Check sheet for the modelled part. Datum: model origin and axes. Units: mm. A direction names the side the tool comes from. Give positions to 0.01 mm unless a question says otherwise; leave off trailing zeros. Loops run counter-clockwise (first coordinate to the right, second up) from the corner with the lowest first, then second, coordinate; pieces in that order, holes last. Notation, with made-up numbers: (-6.75, -12) - (29.25, -12) arc R7 cw to (29.25, -1) - close; hole circle Ø2 at (47.25, 38.5). An arc over 180 degrees is marked (long way). Answer in a Markdown table with one row per item. Add a question column.
(1) Go/stop test with flat-tipped pins: P1, Ø1.9, axis at y = 24.5, z = 3, coming from the -X side; P2, Ø1.9, axis at y = 22, z = 4.5, coming from the +X side; P3, Ø1.9, axis at x = -79, z = 2, coming from the +Y side. Record where each tip stops, or that it passes through.
(2) Sectioned sample at B-B on y = 18.5. Enter the section's corners in (x, z) (3 decimals).
(3) Draft check along X on faces 5 (the face through (-76.325, 15, 3)), 6 (the face through (40, -26.35, 3)), 7 (the face through (10, -23, 3)), 8 (the face through (-30, 23, 3)). Enter one of: released by +X, released by -X, zero draft, split by the parting line, or undercut.
(4) Sectioned sample at A-A on x = 67. Enter the section's corners in (y, z).
(5) Thickness scan on L1, parallel to X at y = 20.5, z = 4.5; L2, parallel to X at y = 19, z = 3.5 (3 decimals); L3, parallel to Y at x = -60, z = 2. Record the ranges inside material, lowest first.
(6) Set-up check for faces 1 (the face through (-80, 10, 3)), 2 (the face through (63, 20, 3)), 3 (the face through (76.325, -15, 3)), 4 (the face through (30, 23, 3)): record each of +Z, -Z, +X, -X, +Y, -Y from which the full face is reachable in a straight line by a thin tool's end or side.
from build123d import *

# Parameters (mm, degrees)
ESQUISSE1_W             = 165.35
ESQUISSE1_H             = 52.7
BOSS_EXTRU_1_DEPTH      = 6.35
ESQUISSE3_W             = 6.35
ESQUISSE3_H             = 16.35
ENL_V_MAT_EXTRU_1_DEPTH = 88.004601171
ESQUISSE5_W             = 20
ESQUISSE5_H             = 6.35
ESQUISSE5_W_2           = 26.325
ENL_V_MAT_EXTRU_2_DEPTH = 88.004601171


with BuildPart() as part:
    # Esquisse1 → Boss.-Extru.1 (new body)
    with BuildSketch(Plane.XY):
        Rectangle(ESQUISSE1_W, ESQUISSE1_H)
    extrude(amount=BOSS_EXTRU_1_DEPTH)

    # Esquisse3 → Enlèv. mat.-Extru.1 (cut, through all)
    with BuildSketch(Plane.XY.offset(6.35)):
        with Locations((-79.5, -18.175)):
            Rectangle(ESQUISSE3_W, ESQUISSE3_H)
        with Locations((-79.5, 18.175)):
            Rectangle(ESQUISSE3_W, ESQUISSE3_H)
    enl_v_mat_extru_1 = extrude(amount=-ENL_V_MAT_EXTRU_1_DEPTH, mode=Mode.SUBTRACT)

    # Symétrie1: Enlèv. mat.-Extru.1 across plane
    add(enl_v_mat_extru_1.mirror(Plane(origin=(0, 0, 0), x_dir=(0, 0, 1), z_dir=(1, 0, 0))), mode=Mode.SUBTRACT)

    # Esquisse5 → Enlèv. mat.-Extru.2 (cut, through all)
    with BuildSketch(Plane.XY.offset(6.35)):
        with Locations((-20, -23.175)):
            Rectangle(ESQUISSE5_W, ESQUISSE5_H)
        with Locations((20, -23.175)):
            Rectangle(ESQUISSE5_W, ESQUISSE5_H)
        with Locations((63.1625, -23.175)):
            Rectangle(ESQUISSE5_W_2, ESQUISSE5_H)
        with Locations((-63.1625, -23.175)):
            Rectangle(ESQUISSE5_W_2, ESQUISSE5_H)
    enl_v_mat_extru_2 = extrude(amount=-ENL_V_MAT_EXTRU_2_DEPTH, mode=Mode.SUBTRACT)

    # Symétrie2: Enlèv. mat.-Extru.2 across plane
    add(enl_v_mat_extru_2.mirror(Plane.ZX), mode=Mode.SUBTRACT)


solid = part.part
Reply:
| question | item | result |
|---|---|---|
| 1 | P1 | x = -50 |
| 1 | P2 | x = 50 |
| 1 | P3 | y = 10 |
| 2 | outline | (-76.325, 0) - (76.325, 0) - (76.325, 6.35) - (-76.325, 6.35) - close |
| 3 | face 5 | released by -X |
| 3 | face 6 | zero draft |
| 3 | face 7 | undercut |
| 3 | face 8 | undercut |
| 4 | outline | (-20, 0) - (20, 0) - (20, 6.35) - (-20, 6.35) - close |
| 5 | L1 | -50 to -30, -10 to 10, 30 to 50 |
| 5 | L2 | -76.325 to 76.325 |
| 5 | L3 | -20 to 20 |
| 6 | face 1 | +Z, -Z, -X, +Y |
| 6 | face 2 | +Z, -Z, +X, +Y |
| 6 | face 3 | +Z, -Z, +X, -Y |
| 6 | face 4 | +Z, -Z, +Y |
